Study the drawing (mm; zero at the part's minimum x, y, z) and answer. A direction names the side the tool comes from. Coordinates: 2 decimals unless noted, no trailing zeros. Loops run counter-clockwise (first coordinate to the right, second up) from the corner with the lowest first, then second, coordinate; pieces in that order, holes last. Notation, with made-up numbers: (64.5, 22) -> (102.5, 22) arc R30 ccw to (102.5, 48) -> close; hole circle Ø5 at (30.25, -2). An arc over 180 degrees is marked (long way). Answer as a JSON object with one key per item and string values. Group by question number.
Q1. The part is cut by section A-A on y = 40.5. Write down the section's boundary in (x, z), and give its area (3 significant figures).
Q2. Determine the mould class of the marked faces 1, 2 and 3 for opening direction Z: released by +Z, released by -Z, zero draft, split by the parting line, or undercut.
Q3. The part is cut by section B-B on z = 39. Write down the section's boundary in (x, y), and give its area (3 significant figures).
Q4. The part is cut by section D-D on z = 17.5. Write down the section's boundary in (x, y).
Q5. Straight lines are drawn through the part: line 1 along X through (y, z) = (16.5, 47.5); line 2 along Y through (x, z) = (13, 44); line 3 along Y through (x, z) = (15, 37). For each, find the intervals that lie inside material, in ascending order. Write a range as [from, to].
Q6. For the marked faces 4, 5, 6, 7 and 8, determine the directions among +Z, -Z, +X, -X, +Y, -Y from which every point of the face is accessible in a straight line to the end or side of a thin tool.
Q7. The part is cut by section C-C on y = 21.5. Write down the section's boundary in (x, z).
Q8. This flat-tipped pin is pushed along its axis until it touches: P1, Ø2, axis at y = 10.5, z = 25, coming from the -X side. Where does it stop, or does it pass through?
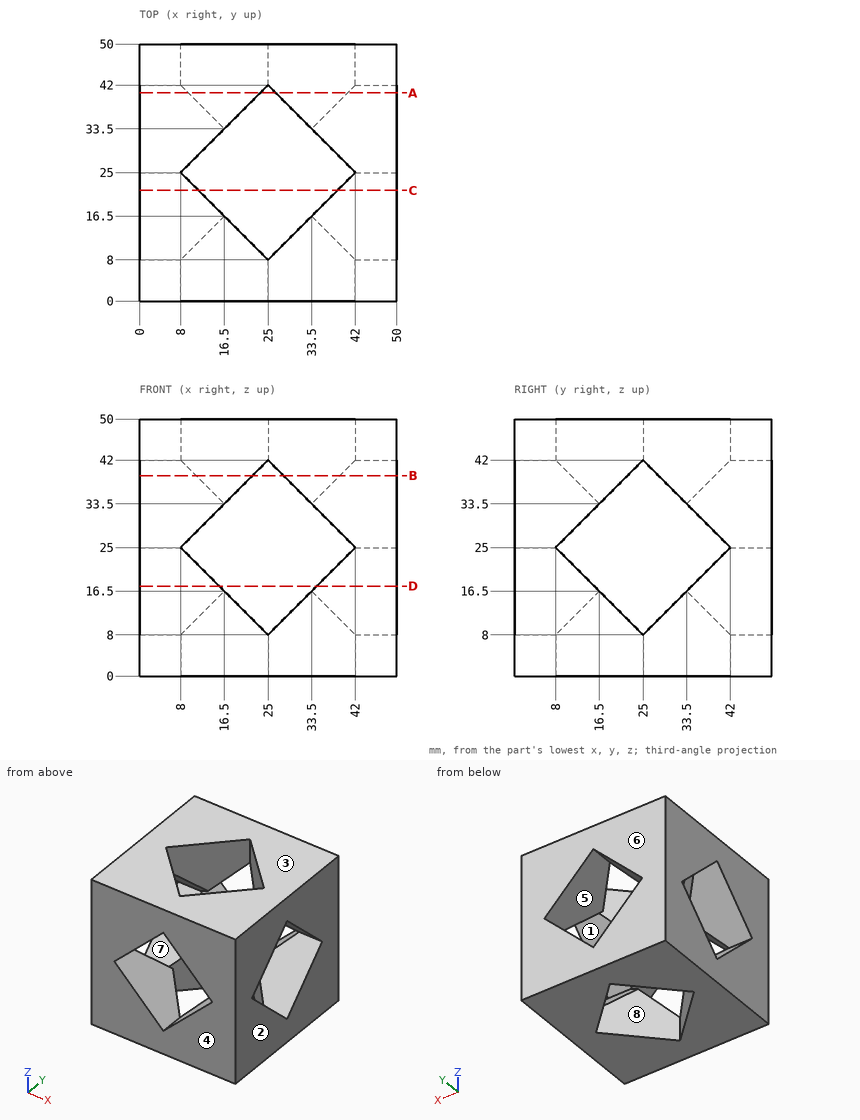
Final values:
{
 "1": {"outline": "(0, 0) -> (23.5, 0) -> (23.5, 9.5) -> (9.5, 23.5) -> (0, 23.5) -> close; (0, 26.5) -> (9.5, 26.5) -> (23.5, 40.5) -> (23.5, 50) -> (0, 50) -> close; (26.5, 0) -> (50, 0) -> (50, 23.5) -> (40.5, 23.5) -> (26.5, 9.5) -> close; (26.5, 40.5) -> (40.5, 26.5) -> (50, 26.5) -> (50, 50) -> (26.5, 50) -> close", "area": "1,820 mm2"},
 "2": {"face 1": "undercut", "face 2": "zero draft", "face 3": "released by +Z"},
 "3": {"outline": "(0, 0) -> (22, 0) -> (22, 11) -> (11, 22) -> (0, 22) -> close; (0, 28) -> (11, 28) -> (22, 39) -> (22, 50) -> (0, 50) -> close; (28, 0) -> (50, 0) -> (50, 22) -> (39, 22) -> (28, 11) -> close; (28, 39) -> (39, 28) -> (50, 28) -> (50, 50) -> (28, 50) -> close", "area": "1,690 mm2"},
 "4": {"outline": "(0, 0) -> (15.5, 0) -> (15.5, 15.5) -> (0, 15.5) -> close; (0, 34.5) -> (15.5, 34.5) -> (15.5, 50) -> (0, 50) -> close; (34.5, 0) -> (50, 0) -> (50, 15.5) -> (34.5, 15.5) -> close; (34.5, 34.5) -> (50, 34.5) -> (50, 50) -> (34.5, 50) -> close"},
 "5": {"line 1": "x = [0, 16.5], [33.5, 50]", "line 2": "y = [0, 20], [30, 50]", "line 3": "y = [0, 18], [32, 50]"},
 "6": {"face 4": "+Z, -Z, +X, -X, -Y", "face 5": "+Y, -Y", "face 6": "+Z, -Z, +X, -X, +Y", "face 7": "+X, -X", "face 8": "+Z, -Z"},
 "7": {"outline": "(0, 0) -> (11.5, 0) -> (11.5, 11.5) -> (0, 11.5) -> close; (0, 38.5) -> (11.5, 38.5) -> (11.5, 50) -> (0, 50) -> close; (38.5, 0) -> (50, 0) -> (50, 11.5) -> (38.5, 11.5) -> close; (38.5, 38.5) -> (50, 38.5) -> (50, 50) -> (38.5, 50) -> close"},
 "8": {"P1": "passes through"}
}
